Could you check a few things on this model? Use its own coordinates, in mm. Face numbers are marked on the shaded views. Give positions to 0.01 mm unless a question says otherwise; leave off trailing zeros. Loops run counter-clockwise (first coordinate to the right, second up) from the corner with the lowest first, then second, coordinate; pieces in that order, holes last. Notation, with made-up numbers: (84, -8) -> (142, -8) arc R20 ccw to (142, 29) -> close; hole circle Ø6 at (22.25, 58). An arc over 180 degrees is marked (long way). Put each result on its own line as item: value.
```python
from build123d import *


with BuildPart() as part:
    # Sketch1 → Revolve1 (revolve)
    with BuildSketch(Plane.XY):
        with BuildLine():
            Line((-6.6802, 0), (-6.6802, -3.175))
            Line((-6.6802, -3.175), (-21.279532816, -50.92726597))
            Line((-21.279532816, -50.92726597), (-25.3996444, -50.92726597))
            Line((-25.3996444, -50.92726597), (-25.3996444, -3.55626597))
            Line((-25.3996444, -3.55626597), (-34.8992444, -3.55626597))
            Line((-34.8992444, -3.55626597), (-34.8992444, 0.76173403))
            Line((-34.8992444, 0.76173403), (-32.8672444, 0.76173403))
            Line((-32.8672444, 0.76173403), (-32.8672444, 4.31773403))
            Line((-32.8672444, 4.31773403), (-34.8992444, 4.31773403))
            Line((-34.8992444, 4.31773403), (-34.8992444, 8.63573403))
            Line((-34.8992444, 8.63573403), (-32.8672444, 8.63573403))
            Line((-32.8672444, 8.63573403), (-32.8672444, 12.19173403))
            Line((-32.8672444, 12.19173403), (-34.8992444, 12.19173403))
            Line((-34.8992444, 12.19173403), (-34.8992444, 16.50973403))
            Line((-34.8992444, 16.50973403), (-33.1466444, 16.50973403))
            Line((-33.1466444, 16.50973403), (-33.1466444, 22.85973403))
            Line((-33.1466444, 22.85973403), (-30.49397, 22.85973403))
            Line((-30.49397, 22.85973403), (-10.691104238, 8.018327423))
            ThreePointArc((-10.691104238, 8.018327423), (-7.73884947, 4.482770557), (-6.6802, 0))
        make_face()
    revolve(axis=Axis((0, 0, 0), (0, -1, 0)))


solid = part.part
```
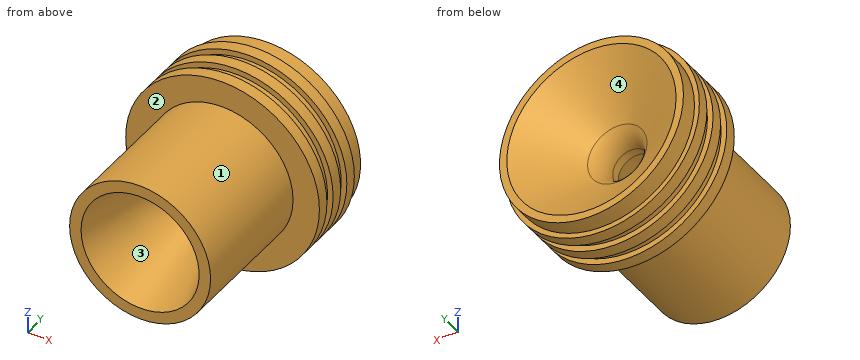
1. If we section it at A-A (y = -11.5): List the corners of the cut face in (x, z) for me.
Recorded:
outline: circle Ø50.8 at (0, 0); hole circle Ø18.45 at (0, 0)
2. I'm going to push flat-ended pins straight in: pin 1 (8 mm diameter, centred on x = 0.5, z = 22, fed in from +Y); pin 2 (6 mm diameter, centred on x = 6.5, y = -14.5, fed in from +Z); pin 3 (1.5 mm diameter, centred on x = -17.5, z = -25, fed in from -Y). Where does each tip first touch, or does it pass through?
Recorded:
pin 1: stops at y = 19.5
pin 2: stops at z = 25.16
pin 3: stops at y = -3.56
3. I need wall thicknesses on line 1 (X direction, y = -0.9, z = 0); line 2 (X direction, y = -37.5, z = -11). Which ranges of each line are inside material? Lowest first, please.
Recorded:
line 1: x = -34.9 to -6.68, 6.68 to 34.9
line 2: x = -22.89 to -13.19, 13.19 to 22.89
4. Thinking about a two-plate mould opening in X: for the marked faces 1, 2, 3 and 4, which applies, pulls with the +X half, pulls with the -X half, needs draft (parallel to the pull), parting line crosses it, or undercut?
Recorded:
face 1: parting line crosses it
face 2: needs draft
face 3: undercut
face 4: undercut
